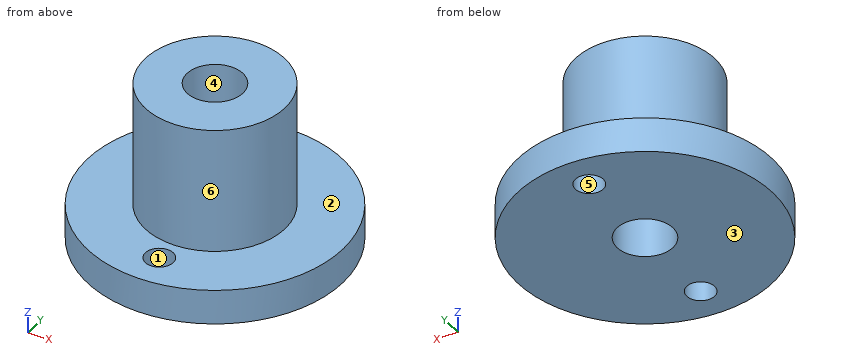
```python
from build123d import *

# Parameters (mm, degrees)
CROQUIS1_R              = 18.25
CROQUIS1_R_2            = 2
SALIENTE_EXTRUIR2_DEPTH = 5
CROQUIS2_R              = 10
SALIENTE_EXTRUIR4_DEPTH = 18
CROQUIS3_R              = 4
CORTAR_EXTRUIR1_DEPTH   = 23


with BuildPart() as part:
    # Croquis1 → Saliente-Extruir2 (new body)
    with BuildSketch(Plane.XY):
        Circle(CROQUIS1_R)
        with Locations((0, 13.2)):
            Circle(CROQUIS1_R_2, mode=Mode.SUBTRACT)
        with Locations(Location((0, -13.2, 0), (0, 0, 180))):
            Circle(CROQUIS1_R_2, mode=Mode.SUBTRACT)
    extrude(amount=-SALIENTE_EXTRUIR2_DEPTH)

    # Croquis2 → Saliente-Extruir4 (add)
    with BuildSketch(Plane.XY):
        Circle(CROQUIS2_R)
    extrude(amount=SALIENTE_EXTRUIR4_DEPTH)

    # Croquis3 → Cortar-Extruir1 (cut)
    with BuildSketch(Plane.XY.offset(18)):
        Circle(CROQUIS3_R)
    extrude(amount=-CORTAR_EXTRUIR1_DEPTH, mode=Mode.SUBTRACT)


solid = part.part
```
Build history of the part. All positions in model axes, mm. Face numbers are marked on the shaded views. A direction names the side the tool comes from. Round coordinates to 2 decimals unless told otherwise and drop trailing zeros. Write each loop counter-clockwise with the first axis right and the second up, starting at its lowest first coordinate (ties: lowest second). Pieces come first, ordered by that corner, then holes.
1) Band-saw the part on C-C, the plane z = 1.75. List the corners of the cut face in (x, y), and give its area (3 significant figures).
2) 3-axis set-ups, long thin cutter, end or side, ignore diameter. For the marked faces 1 and 2: which of +Z, -Z, +X, -X, +Y, -Y reach the whole face in a straight line?
3) Pin check, flat tips, straight feed: pin 1 (5 mm diameter, centred on y = -7.5, z = 0, fed in from +X); pin 2 (3 mm diameter, centred on y = 8.5, z = 12, fed in from -X); pin 3 (1 mm diameter, centred on y = 7, z = 8.5, fed in from -X). Stop position of each tip, or through.
4) Mould opens along X. For the marked faces 3, 4, 5 and 6 say: +X half, -X half, draft (parallel to the pull), parting line (faces both ways), or undercut.
5) Band-saw the part on D-D, the plane z = -3.5. List the corners of the cut face in (x, y).
6) Band-saw the part on A-A, the plane y = 0. List the corners of the cut face in (x, z), and give its area (4 significant figures).
7) Band-saw the part on B-B, the plane x = 0. List the corners of the cut face in (y, z).
8) Drill centre lines: probe 1 along Y at (x, z) = (0, -1.6); probe 2 along Y at (x, z) = (0, 9); probe 3 along Z at (x, y) = (10.5, 1.5). Where is each one in solid material? Low to high.
Ans:
1. outline: circle Ø20 at (0, 0); hole circle Ø8 at (0, 0)
1. area: 264 mm2
2. face 1: +Z, -Z
2. face 2: +Z
3. pin 1: stops at x = 17.55
3. pin 2: stops at x = -7.14
3. pin 3: stops at x = -7.6
4. face 3: draft
4. face 4: undercut
4. face 5: undercut
4. face 6: parting line
5. outline: circle Ø36.5 at (0, 0); hole circle Ø8 at (0, 0); hole circle Ø4 at (0, -13.2); hole circle Ø4 at (0, 13.2)
6. outline: (-18.25, -5) - (-4, -5) - (-4, 18) - (-10, 18) - (-10, 0) - (-18.25, 0) - close; (4, -5) - (18.25, -5) - (18.25, 0) - (10, 0) - (10, 18) - (4, 18) - close
6. area: 358.5 mm2
7. outline: (-18.25, -5) - (-15.2, -5) - (-15.2, 0) - (-18.25, 0) - close; (-11.2, -5) - (-4, -5) - (-4, 18) - (-10, 18) - (-10, 0) - (-11.2, 0) - close; (4, -5) - (11.2, -5) - (11.2, 0) - (10, 0) - (10, 18) - (4, 18) - close; (15.2, -5) - (18.25, -5) - (18.25, 0) - (15.2, 0) - close
8. probe 1: y = -18.25 to -15.2, -11.2 to -4, 4 to 11.2, 15.2 to 18.25
8. probe 2: y = -10 to -4, 4 to 10
8. probe 3: z = -5 to 0
